from build123d import *

# Parameters (mm, degrees)
F0_W     = 35
F0_H     = 6
F1_DEPTH = 25
F3_DEPTH = 25
F4_DEPTH = 25


# Not quite as in the source:
# - a feature names something its author has since deleted; it is built from what else it names


with BuildPart() as f1:
    # F0 (on Top) → F1 (new body)
    with BuildSketch(Plane.XY):
        with Locations((-28.5, -30)):
            Rectangle(F0_W, F0_H)
        Polygon((-5, 3), (-11, 3), (-11, -3), (-11, -27), (-11, -33), (-5, -33), (-5, -3), align=None)
    extrude(amount=F1_DEPTH)

    # F2 (on face) → F3 (cut)
    with BuildSketch(Plane(origin=(0, -27, 0), x_dir=(-1, 0, 0), z_dir=(0, 1, 0))):
        with BuildLine():
            ThreePointArc((31, 8), (34.1819805153, 9.3180194847), (35.5, 12.5))
            ThreePointArc((35.5, 12.5), (34.1819805153, 15.6819805153), (31, 17))
            ThreePointArc((31, 17), (26.5, 12.5), (31, 8))
        make_face()
    extrude(amount=-F3_DEPTH, mode=Mode.SUBTRACT)

    # F2 (on face) → F4 (cut)
    with BuildSketch(Plane(origin=(0, -27, 0), x_dir=(-1, 0, 0), z_dir=(0, 1, 0))):
        with BuildLine():
            ThreePointArc((31, 17), (34.1819805153, 15.6819805153), (35.5, 12.5))
            ThreePointArc((35.5, 12.5), (34.1819805153, 9.3180194847), (31, 8))
            Line((31, 8), (46, 8))
            Line((46, 8), (46, 17))
            Line((46, 17), (31, 17))
        make_face()
    extrude(amount=-F4_DEPTH, mode=Mode.SUBTRACT)


solid = f1.part
Geometry: final body of the model. Coordinates: model frame, mm. A direction names the side the tool comes from. Round coordinates to 2 decimals unless told otherwise and drop trailing zeros. Loops run counter-clockwise (first coordinate to the right, second up) from the corner with the lowest first, then second, coordinate; pieces in that order, holes last.
Q1. Section A-A on x = -39. Return loops of the section in (y, z).
Q2. Section B-B on z = 22.75. Return loops of the section in (x, y).
Q3. Pin query (flat end, axial travel): P1, Ø1.5, axis at x = -39, z = 8, coming from the +Y side; P2, Ø8, axis at y = -3.5, z = 9.5, coming from the -X side. Return the tip coordinate at first contact, or that it passes through.
Q4. Material intervals for L1, parallel to X at y = -21, z = 23.25; L2, parallel to Y at x = -19, z = 15; L3, parallel to Z at x = -42, y = -27.5, sorted ascending.
Q5. Pull-direction query (Z, two-part tool) for faces 4 (the flat face through (-25, -27, 12)), 5 (the flat face through (-39, -30, 17)), 6 (the flat face through (-20, -28, 25)), 7 (the cylindrical face through (-26.5, -30, 12.6)); classes: released by +Z, released by -Z, zero draft, split by the parting line, or undercut.
Q6. Section D-D on z = 12.5. Return loops of the section in (x, y), plus the area to 3 significant figures.
Q7. Section C-C on y = -6.5. Return loops of the section in (x, z), plus the area to 3 significant figures.
Q8. Access query for faces 1 (the flat face through (-8, 3, 12)), 2 (the flat face through (-11, -12, 12)), 3 (the flat face through (-38, -30, 8)). Directions: +Z, -Z, +X, -X, +Y, -Y. A direction counts if a zero-diameter tool reaches every point of the face in a straight line with its end or side. Return the directions, or none.
Evaluation:
1. outline: (-33, 0) - (-27, 0) - (-27, 8) - (-33, 8) - close; (-33, 17) - (-27, 17) - (-27, 25) - (-33, 25) - close
2. outline: (-46, -33) - (-5, -33) - (-5, 3) - (-11, 3) - (-11, -27) - (-46, -27) - close
3. P1: stops at y = -27
3. P2: stops at x = -11
4. L1: x = -11 to -5
4. L2: y = -33 to -27
4. L3: z = 0 to 8, 17 to 25
5. face 4: zero draft
5. face 5: undercut
5. face 6: released by +Z
5. face 7: undercut
6. outline: (-26.5, -33) - (-5, -33) - (-5, 3) - (-11, 3) - (-11, -27) - (-26.5, -27) - close
6. area: 309 mm2
7. outline: (-11, 0) - (-5, 0) - (-5, 25) - (-11, 25) - close
7. area: 150 mm2
8. face 1: +Z, -Z, +X, -X, +Y
8. face 2: +Z, -Z, -X, +Y
8. face 3: -X, +Y, -Y
